```python
from build123d import *

# Parameters (mm, degrees)
SKETCH1_W           = 25
SKETCH1_H           = 38
BOSS_EXTRUDE1_DEPTH = 12
SKETCH3_W           = 25
SKETCH3_H           = 12
BOSS_EXTRUDE2_DEPTH = 5.5
SKETCH5_W           = 25
SKETCH5_H           = 5
BOSS_EXTRUDE3_DEPTH = 21
SKETCH6_R           = 1.25
CUT_EXTRUDE1_DEPTH  = 10
SKETCH7_W           = 75
SKETCH7_H           = 49
BOSS_EXTRUDE4_DEPTH = 10
SKETCH8_W           = 65
SKETCH8_H           = 12
CUT_EXTRUDE2_DEPTH  = 3.5
SKETCH11_W          = 25
SKETCH11_H          = 39
CUT_EXTRUDE4_DEPTH  = 2.5
SKETCH12_W          = 75
SKETCH12_H          = 10
BOSS_EXTRUDE6_DEPTH = 20.32
SKETCH15_W          = 69.32
SKETCH15_H          = 10
BOSS_EXTRUDE7_DEPTH = 32.5
SKETCH16_W          = 69.32
SKETCH16_H          = 10
BOSS_EXTRUDE8_DEPTH = 32.5
SKETCH19_W          = 12
SKETCH19_H          = 3.5
CUT_EXTRUDE6_DEPTH  = 38.5
SKETCH23_W          = 102.5
SKETCH23_H          = 3.5
CUT_EXTRUDE7_DEPTH  = 5
SKETCH24_W          = 102.5
SKETCH24_H          = 3.5
CUT_EXTRUDE8_DEPTH  = 5
SKETCH25_W          = 37.5
SKETCH25_H          = 69.32
CUT_EXTRUDE9_DEPTH  = 3.5


with BuildPart() as part:
    # Sketch1 → Boss-Extrude1 (new body)
    with BuildSketch(Plane(origin=(0, 0, 0), x_dir=(1, 0, 0), z_dir=(0, 1, 0))):
        with Locations((12.5, 19)):
            Rectangle(SKETCH1_W, SKETCH1_H)
    extrude(amount=BOSS_EXTRUDE1_DEPTH)

    # Sketch3 → Boss-Extrude2 (add)
    with BuildSketch(Plane.XY):
        with Locations((12.5, 6)):
            Rectangle(SKETCH3_W, SKETCH3_H)
    boss_extrude2 = extrude(amount=BOSS_EXTRUDE2_DEPTH)

    # Sketch5 → Boss-Extrude3 (add)
    with BuildSketch(Plane.XZ):
        with Locations((12.5, 3)):
            Rectangle(SKETCH5_W, SKETCH5_H)
    boss_extrude3 = extrude(amount=BOSS_EXTRUDE3_DEPTH)

    # Sketch6 → Cut-Extrude1 (cut)
    with BuildSketch(Plane.XY.offset(5.5)):
        with Locations((3, -16.5)):
            Circle(SKETCH6_R)
        with Locations((22.59, -16.5)):
            Circle(SKETCH6_R)
        with Locations((22.59, -3.53)):
            Circle(SKETCH6_R)
        with Locations((3, -3.53)):
            Circle(SKETCH6_R)
    cut_extrude1 = extrude(amount=-CUT_EXTRUDE1_DEPTH, mode=Mode.SUBTRACT)

    # Mirror1: Boss-Extrude2, Boss-Extrude3, Cut-Extrude1 across plane
    add(boss_extrude2.mirror(Plane.XY.offset(-19)))
    add(boss_extrude3.mirror(Plane.XY.offset(-19)))
    add(cut_extrude1.mirror(Plane.XY.offset(-19)), mode=Mode.SUBTRACT)

    # Sketch7 → Boss-Extrude4 (add)
    with BuildSketch(Plane(origin=(0, 12, 0), x_dir=(1, 0, 0), z_dir=(0, 1, 0))):
        with Locations((12.5, 19)):
            Rectangle(SKETCH7_W, SKETCH7_H)
    extrude(amount=BOSS_EXTRUDE4_DEPTH)

    # Sketch8 → Cut-Extrude2 (cut)
    with BuildSketch(Plane(origin=(0, 22, 0), x_dir=(1, 0, 0), z_dir=(0, 1, 0))):
        with Locations((12.5, 29)):
            Rectangle(SKETCH8_W, SKETCH8_H)
    extrude(amount=-CUT_EXTRUDE2_DEPTH, mode=Mode.SUBTRACT)

    # Sketch11 → Cut-Extrude4 (cut)
    with BuildSketch(Plane.XZ):
        with Locations((12.5, -19)):
            Rectangle(SKETCH11_W, SKETCH11_H)
    extrude(amount=-CUT_EXTRUDE4_DEPTH, mode=Mode.SUBTRACT)

    # Sketch12 → Boss-Extrude6 (add)
    with BuildSketch(Plane(origin=(0, 0, -43.5), x_dir=(-1, 0, 0), z_dir=(0, 0, -1))):
        with Locations((-12.5, 17)):
            Rectangle(SKETCH12_W, SKETCH12_H)
    extrude(amount=BOSS_EXTRUDE6_DEPTH)

    # Sketch15 → Boss-Extrude7 (add)
    with BuildSketch(Plane(origin=(50, 0, 0), x_dir=(0, 0, -1), z_dir=(1, 0, 0))):
        with Locations((29.16, 17)):
            Rectangle(SKETCH15_W, SKETCH15_H)
    extrude(amount=BOSS_EXTRUDE7_DEPTH)

    # Sketch16 → Boss-Extrude8 (add)
    with BuildSketch(Plane.ZY.offset(25)):
        with Locations((-29.16, 17)):
            Rectangle(SKETCH16_W, SKETCH16_H)
    extrude(amount=BOSS_EXTRUDE8_DEPTH)

    # Sketch19 → Cut-Extrude6 (cut, through all)
    with BuildSketch(Plane.ZY.offset(-45)):
        with Locations((-29, 20.25)):
            Rectangle(SKETCH19_W, SKETCH19_H)
    extrude(amount=-CUT_EXTRUDE6_DEPTH, mode=Mode.SUBTRACT)

    # Sketch23 → Cut-Extrude7 (cut)
    with BuildSketch(Plane.XY.offset(-35)):
        with Locations((31.25, 20.25)):
            Rectangle(SKETCH23_W, SKETCH23_H)
    extrude(amount=-CUT_EXTRUDE7_DEPTH, mode=Mode.SUBTRACT)

    # Sketch24 → Cut-Extrude8 (cut)
    with BuildSketch(Plane(origin=(0, 0, -23), x_dir=(-1, 0, 0), z_dir=(0, 0, -1))):
        with Locations((-31.25, 20.25)):
            Rectangle(SKETCH24_W, SKETCH24_H)
    extrude(amount=-CUT_EXTRUDE8_DEPTH, mode=Mode.SUBTRACT)

    # Sketch25 → Cut-Extrude9 (cut)
    with BuildSketch(Plane(origin=(0, 22, 0), x_dir=(1, 0, 0), z_dir=(0, 1, 0))):
        with Locations((63.75, 29.16)):
            Rectangle(SKETCH25_W, SKETCH25_H)
    extrude(amount=-CUT_EXTRUDE9_DEPTH, mode=Mode.SUBTRACT)


solid = part.part
```
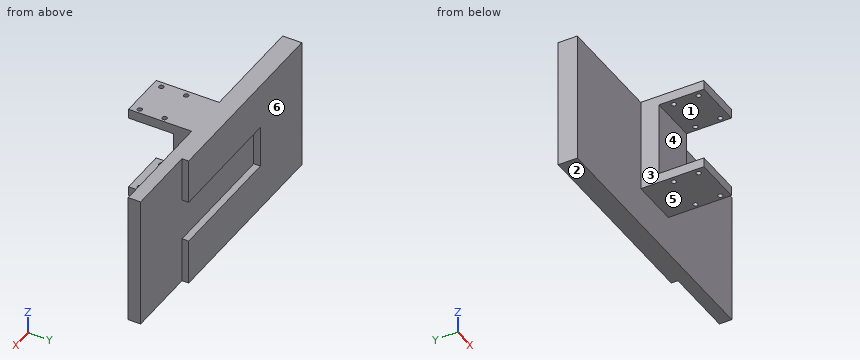
Part model, mm, in its own coordinate system. Face numbers are marked on the shaded views. A direction names the side the tool comes from. Round coordinates to 2 decimals unless told otherwise and drop trailing zeros. Loops run counter-clockwise (first coordinate to the right, second up) from the corner with the lowest first, then second, coordinate; pieces in that order, holes last. Notation, with made-up numbers: (6, 36) -> (52, 36) arc R32 cw to (52, 62) -> close; hole circle Ø5 at (44.5, 29). An arc over 180 degrees is marked (long way). Use one line per item in the form item = value. Start each with the question number.
Item 1: Band-saw the part on C-C (x = -23). List the corners of the cut face in (y, z), plus the area to 3 significant figures.
Item 2: Band-saw the part on D-D (z = -3.5). List the corners of the cut face in (x, y), plus the area to 3 significant figures.
Item 3: Band-saw the part on A-A (y = 0). List the corners of the cut face in (x, z).
Item 4: Two-plate mould, pull along Z, no slides. Class the marked faces 4, 5 and 6: released by +Z, released by -Z, zero draft, split by the parting line, or undercut.
Item 5: Drill centre lines: line 1 along Y through (x, z) = (22.59, -42.05); line 2 along X through (y, z) = (-3.53, -40.6); line 3 along X through (y, z) = (-16, -41). Where is each one in solid material? Low to high.
Item 6: Drop flat-ended pins along their axis: pin 1 Ø4 at (x, y) = (3, -16.5) entering from -Z; pin 2 Ø1.8 at (y, z) = (19.5, -48) entering from +X; pin 3 Ø10 at (x, z) = (62.5, -36) entering from -Y. Give the stop position or say it passes through.
Item 7: Tool access for the marked faces 1, 2 and 3: list every direction of +Z, -Z, +X, -X, +Y, -Y with a clear straight run to the whole face (end or side of a thin tool).
Item 8: Band-saw the part on B-B (z = -32). List the corners of the cut face in (x, y), plus the area to 3 significant figures.
Data:
q1.outline = (12, -63.82) -> (22, -63.82) -> (22, 5.5) -> (12, 5.5) -> close
q1.area = 693 mm^2
q2.outline = (-57.5, 12) -> (0, 12) -> (0, 2.5) -> (25, 2.5) -> (25, 12) -> (82.5, 12) -> (82.5, 18.5) -> (45, 18.5) -> (45, 22) -> (-57.5, 22) -> close
q2.area = 1,510 mm^2
q3.outline = (0, -43.5) -> (25, -43.5) -> (25, -38.5) -> (0, -38.5) -> close; (0, 0.5) -> (25, 0.5) -> (25, 5.5) -> (0, 5.5) -> close
q4.face_4 = undercut
q4.face_5 = released by -Z
q4.face_6 = zero draft
q5.line_1 = -21 to -17.75, -15.25 to -4.78, -2.28 to 22
q5.line_2 = 0 to 1.75, 4.25 to 21.34, 23.84 to 25
q5.line_3 = 0 to 1.85, 4.15 to 21.44, 23.74 to 25
q6.pin_1 = -43.5
q6.pin_2 = 45
q6.pin_3 = 12
q7.face_1 = +X, -X, -Y
q7.face_2 = -Z, +X, -X, +Y, -Y
q7.face_3 = +Z, -Z, -X, -Y
q8.outline = (-57.5, 12) -> (0, 12) -> (0, 2.5) -> (25, 2.5) -> (25, 12) -> (82.5, 12) -> (82.5, 18.5) -> (-20, 18.5) -> (-20, 22) -> (-57.5, 22) -> close
q8.area = 1,280 mm^2
